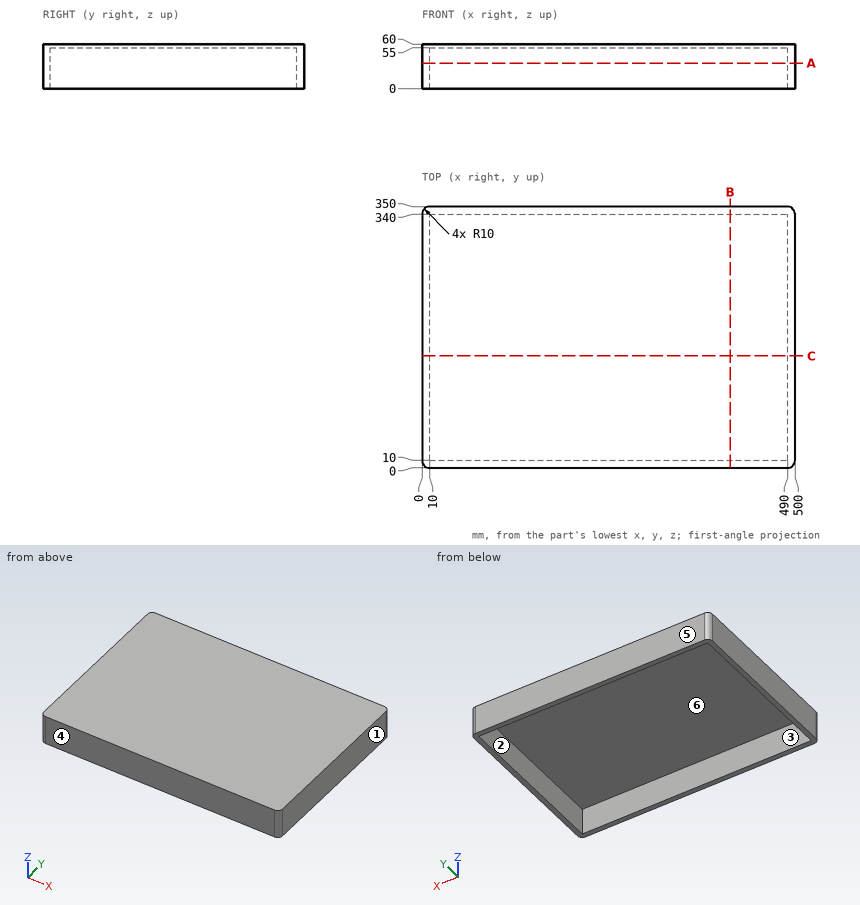
For this review, use the dimensioned drawing (mm, ordinates from the lowest corner) and the shaded views. A direction names the side the tool comes from. Coordinates: 2 decimals unless noted, no trailing zeros. Write each loop counter-clockwise with the first axis right and the second up, starting at its lowest first coordinate (ties: lowest second). Pieces come first, ordered by that corner, then holes. Notation, with made-up numbers: (47, 13.25) - (76, 13.25) arc R20 ccw to (76, 37.25) - close; hole circle Ø8 at (-28.5, 56.5). An arc over 180 degrees is marked (long way). Answer as a JSON object with one key per item and string values. Group by question number.
1. Machinability: for the marked faces 5 and 6, which of the approach directions +Z, -Z, +X, -X, +Y, -Y give a long, thin tool a straight path to every point of the face, cutting with its end or side? Answer none if there is none.
2. Add section B-B (x = 413). Give the boundary of the cut face in (y, z).
3. Mouldability with a two-part tool opening along Y and no side actions: class the marked faces 1, 2, 3 and 4 as pulls with the +Y half, pulls with the -Y half, needs draft (parallel to the pull), parting line crosses it, or undercut.
4. Add section C-C (y = 150). Give the boundary of the cut face in (x, z), plus the area to 3 significant figures.
5. Clearance check with a flat-ended pin moving along its axis: pin 1 Ø10 at (x, y) = (445, 284.5) entering from -Z. State where the tip first meets the part, or that it passes through.
6. To check wall thickness, follow probe 1 along Y at (x, z) = (66, 51); probe 2 along X at (y, z) = (147, 13.5); probe 3 along Z at (x, y) = (42, 231.5). State the ranges of each line that lie inside material, in increasing order.
7. Add section A-A (z = 34.5). Give the boundary of the cut face in (x, y), plus the area to 3 significant figures.
Findings:
{
 "1": {"face 5": "+Z, -Z, +X, -X, +Y", "face 6": "-Z"},
 "2": {"outline": "(0, 0) - (10, 0) - (10, 55) - (340, 55) - (340, 0) - (350, 0) - (350, 60) - (0, 60) - close"},
 "3": {"face 1": "needs draft", "face 2": "undercut", "face 3": "undercut", "face 4": "pulls with the -Y half"},
 "4": {"outline": "(0, 0) - (10, 0) - (10, 55) - (490, 55) - (490, 0) - (500, 0) - (500, 60) - (0, 60) - close", "area": "3,600 mm²"},
 "5": {"pin 1": "z = 55"},
 "6": {"probe 1": "0 to 10, 340 to 350", "probe 2": "0 to 10, 490 to 500", "probe 3": "55 to 60"},
 "7": {"outline": "(0, 10) arc R10 ccw to (10, 0) - (490, 0) arc R10 ccw to (500, 10) - (500, 340) arc R10 ccw to (490, 350) - (10, 350) arc R10 ccw to (0, 340) - close; hole (10, 10) - (490, 10) - (490, 340) - (10, 340) - close", "area": "16,500 mm²"}
}
